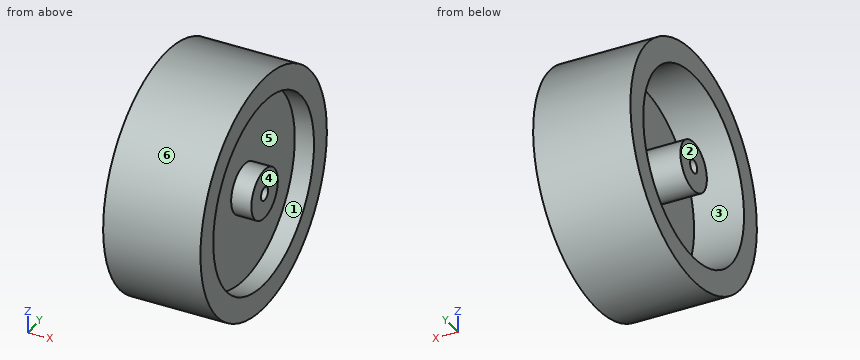
from build123d import *

# Parameters (mm, degrees)
SKETCH2_R               = 32.5
BOSS_EXTRUDE1_DEPTH     = 26.6
SKETCH3_R               = 25.9
CUT_EXTRUDE2_DEPTH      = 5.264
CUT_EXTRUDE3_START      = -13.646
SKETCH4_R               = 25.9
CUT_EXTRUDE3_DEPTH      = 13.646
SKETCH5_R               = 6.8
BOSS_EXTRUDE2_DEPTH     = 13.646
BOSS_EXTRUDE3_START     = 5.518
SKETCH6_R               = 6.8
BOSS_EXTRUDE3_DEPTH     = 5.518
CUT_EXTRUDE4_DEPTH      = 28.702
CUT_EXTRUDE4_DEPTH_BACK = 38.03
SKETCH7_R               = 1.83
SCALE1_SCALE            = 0.8
SCALE2_SCALE            = 0.8
SCALE3_SCALE            = 0.8


with BuildPart() as part:
    # Sketch2 → Boss-Extrude1 (new body)
    with BuildSketch(Plane(origin=(0, 0, 0), x_dir=(0, 0, -1), z_dir=(1, 0, 0))):
        Circle(SKETCH2_R)
    extrude(amount=BOSS_EXTRUDE1_DEPTH)

    # Sketch3 → Cut-Extrude2 (cut)
    with BuildSketch(Plane(origin=(26.6, 0, 0), x_dir=(0, 0, -1), z_dir=(1, 0, 0))):
        Circle(SKETCH3_R)
    extrude(amount=-CUT_EXTRUDE2_DEPTH, mode=Mode.SUBTRACT)

    # Sketch4 → Cut-Extrude3 (cut)
    with BuildSketch(Plane.ZY.offset(CUT_EXTRUDE3_START)):
        with Locations(Location((0, 0, 0), (0, 0, 180))):
            Circle(SKETCH4_R)
    extrude(amount=CUT_EXTRUDE3_DEPTH, mode=Mode.SUBTRACT)

    # Sketch5 → Boss-Extrude2 (add)
    with BuildSketch(Plane.ZY.offset(-13.646)):
        with Locations(Location((0, 0, 0), (0, 0, 180))):
            Circle(SKETCH5_R)
    extrude(amount=BOSS_EXTRUDE2_DEPTH)

    # Sketch6 → Boss-Extrude3 (add)
    with BuildSketch(Plane(origin=(21.336, 0, 0), x_dir=(0, 0, -1), z_dir=(1, 0, 0)).offset(BOSS_EXTRUDE3_START)):
        Circle(SKETCH6_R)
    extrude(amount=-BOSS_EXTRUDE3_DEPTH)

    # Sketch7 → Cut-Extrude4 (cut, two sides: drawn at the far end of the back side and taken through both)
    with BuildSketch(Plane(origin=(26.854, 0, 0), x_dir=(0, 0, -1), z_dir=(1, 0, 0)).offset(-CUT_EXTRUDE4_DEPTH_BACK)):
        with Locations(Location((0, 0, 0), (0, 0, 180))):
            Circle(SKETCH7_R)
    extrude(amount=CUT_EXTRUDE4_DEPTH + CUT_EXTRUDE4_DEPTH_BACK, mode=Mode.SUBTRACT)


with BuildPart() as part_1:
    # Scale1: scaled about (14.550993836, 0, 0)
    add(part.part.scale(SCALE1_SCALE).moved(Location((2.910198767, 0, 0))))


with BuildPart() as part_2:
    # Scale2: scaled about (14.550993836, 0, 0)
    add(part_1.part.scale(SCALE2_SCALE).moved(Location((2.910198767, 0, 0))))


with BuildPart() as part_3:
    # Scale3: scaled about (14.550993836, 0, 0)
    add(part_2.part.scale(SCALE3_SCALE).moved(Location((2.910198767, 0, 0))))


solid = part_3.part
Input: part model. Units: mm. Frame: model coordinates. Face numbers are marked on the shaded views. A direction names the side the tool comes from. Give positions to 0.01 mm unless a question says otherwise; leave off trailing zeros. Write each loop counter-clockwise with the first axis right and the second up, starting at its lowest first coordinate (ties: lowest second). Pieces come first, ordered by that corner, then holes.
Q1. First-contact query: P1, Ø3, axis at y = -9, z = -3, coming from the +X side; P2, Ø16.5, axis at y = -7.5, z = -1, coming from the +X side; P3, Ø5, axis at x = 9.5, z = 8, coming from the -Y side; P4, Ø1.5, axis at y = 0, z = 0, coming from the -X side. Flat tips, straight axial feed; report the tip coordinate or a pass-through.
Q2. Material intervals for probe 1 along Y at (x, z) = (11, 0); probe 2 along Y at (x, z) = (16.75, 0); probe 3 along X at (y, z) = (-4, -4), sorted ascending.
Q3. Section C-C, the plane x = 19.5. Output: boundary loops of the cut face in (y, z), plus the area to 3 significant figures.
Q4. Set-up query: the marked faces 1, 2 and 3. Return all of +Z, -Z, +X, -X, +Y, -Y with unobstructed straight access to the full face (end or side cutting, diameter ignored); none if empty.
Q5. Section D-D, the plane z = 12.5. Output: boundary loops of the cut face in (x, y).
Q6. Section A-A, the plane z = 0. Output: boundary loops of the cut face in (x, y).
Q7. Pull-direction query (Y, two-part tool) for the marked faces 4, 5 and 6; classes: pulls with the +Y half, pulls with the -Y half, needs draft (parallel to the pull), parting line crosses it, or undercut.
Filled in:
1. P1: stops at x = 18.02
1. P2: stops at x = 20.85
1. P3: stops at y = -15.7
1. P4: passes through
2. probe 1: y = -16.64 to -13.26, -3.48 to -0.94, 0.94 to 3.48, 13.26 to 16.64
2. probe 2: y = -16.64 to -0.94, 0.94 to 16.64
2. probe 3: x = 14.09 to 18.02
3. outline: circle Ø33.28 at (0, 0); circle Ø6.96 at (0, 0); hole circle Ø26.52 at (0, 0); hole circle Ø1.87 at (0, 0)
3. area: 353 mm2
4. face 1: +X
4. face 2: +Z, -Z, -X, +Y, -Y
4. face 3: -X
5. outline: (7.1, -10.98) - (20.72, -10.98) - (20.72, -4.43) - (18.02, -4.43) - (18.02, 4.43) - (20.72, 4.43) - (20.72, 10.98) - (7.1, 10.98) - (7.1, 4.43) - (14.09, 4.43) - (14.09, -4.43) - (7.1, -4.43) - close
6. outline: (7.1, -16.64) - (20.72, -16.64) - (20.72, -13.26) - (18.02, -13.26) - (18.02, -3.48) - (20.85, -3.48) - (20.85, -0.94) - (7.1, -0.94) - (7.1, -3.48) - (14.09, -3.48) - (14.09, -13.26) - (7.1, -13.26) - close; (7.1, 0.94) - (20.85, 0.94) - (20.85, 3.48) - (18.02, 3.48) - (18.02, 13.26) - (20.72, 13.26) - (20.72, 16.64) - (7.1, 16.64) - (7.1, 13.26) - (14.09, 13.26) - (14.09, 3.48) - (7.1, 3.48) - close
7. face 4: needs draft
7. face 5: undercut
7. face 6: parting line crosses it
